Design review of the part built by this model. Coordinates are the model's own, in mm. Face numbers are marked on the shaded views. A direction names the side the tool comes from. Coordinates: 2 decimals unless noted, no trailing zeros. Write each loop counter-clockwise with the first axis right and the second up, starting at its lowest first coordinate (ties: lowest second). Pieces come first, ordered by that corner, then holes. Notation, with made-up numbers: (48, -34) - (96, -34) arc R32 cw to (96, -1) - close; hole circle Ø6 at (51.5, 58). An arc over 180 degrees is marked (long way). Answer as a JSON object with one key per item and string values.
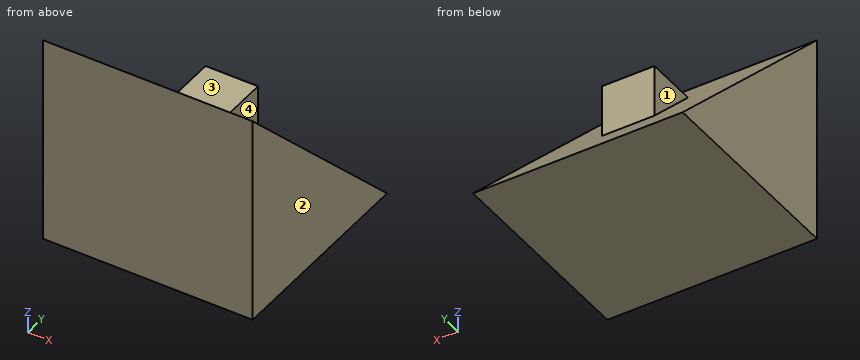
```python
from build123d import *

# Parameters (mm, degrees)
F1_DEPTH = 20
F2_DEPTH = 5


with BuildPart() as f1:
    # F0 (on Right) → F1 (new body, symmetric)
    with BuildSketch(Plane.YZ):
        Polygon((-5, 5), (-20, 20), (-20, -20), (20, -20), (5, -5), (-5, -5), align=None)
        Polygon((5, -5), (-5, 5), (-5, -5), align=None)
    extrude(amount=F1_DEPTH, both=True)

    # F0 (on Right) → F2 (join, symmetric)
    with BuildSketch(Plane.YZ):
        Polygon((5, 5), (-5, 5), (5, -5), align=None)
    extrude(amount=F2_DEPTH, both=True)


solid = f1.part
```
(1) Take a section at B-B, the plane x = -3.5. Write out the cut boundary in (y, z).
Solved:
{"outline": "(-20, -20) - (20, -20) - (5, -5) - (5, 5) - (-5, 5) - (-20, 20) - close"}
(2) For pin 1 (3 mm diameter, centred on x = -2, z = 0.5, fed in from +Y); pin 2 (8 mm diameter, centred on x = 2, y = -2, fed in from +Z); pin 3 (10 mm diameter, centred on x = -7, y = 7.5, fed in from +Z), all flat-tipped, find the tip position at first contact; note any pin that passes through.
Solved:
{"pin 1": "stops at y = 5", "pin 2": "stops at z = 6", "pin 3": "stops at z = 5"}
(3) Tool access review of the marked faces 1, 2, 3 and 4: name each direction out of +Z, -Z, +X, -X, +Y, -Y from which nothing blocks a thin tool from reaching the whole face with its end or side.
Solved:
{"face 1": "+Z, -X, +Y", "face 2": "+Z, -Z, +X, +Y, -Y", "face 3": "+Z, +X, -X, +Y", "face 4": "+Z, +X, +Y"}
(4) Take a section at A-A, the plane z = 1. Write out the cut boundary in (x, y), and give its area (3 significant figures).
Solved:
{"outline": "(-20, -20) - (20, -20) - (20, -1) - (5, -1) - (5, 5) - (-5, 5) - (-5, -1) - (-20, -1) - close", "area": "820 mm^2"}
(5) Take a section at D-D, the plane y = 8. Write out the cut boundary in (x, z), and give its area (3 significant figures).
Solved:
{"outline": "(-20, -20) - (20, -20) - (20, -8) - (-20, -8) - close", "area": "480 mm^2"}
(6) Take a section at C-C, the plane y = -7.5. Write out the cut boundary in (x, z).
Solved:
{"outline": "(-20, -20) - (20, -20) - (20, 7.5) - (-20, 7.5) - close"}
(7) To check wall thickness, follow line 1 (Y direction, x = 3, z = -1.5); line 2 (Y direction, x = -13, z = 15). State the ranges of each line that lie inside material, in increasing order. Write a range as from..to.
Solved:
{"line 1": "y = -20..5", "line 2": "y = -20..-15"}
